from build123d import *
from OCP.BRepFilletAPI import BRepFilletAPI_MakeChamfer

# Parameters (mm, degrees)
DOWELSUPPORT_DEPTH       = 1.905
DOWELSUPPORT_DEPTH_BACK  = 1.27
SKETCH3_R                = 3.81
SKETCH5_W                = 9.525
SKETCH5_H                = 31.75
SLIDERDOWELSUPPORT_DEPTH = 1.27
STRINGDOWELSUPPORT_DEPTH = 1.27
SKETCH9_W                = 6.35
SKETCH9_H                = 3
TABSUPPORT_DEPTH         = 1.27
INTERSUPPORT_DEPTH       = 1.27
DOWELHOLES_DEPTH         = 36.095686544
DOWELHOLES_DEPTH_BACK    = 36.095686544
SKETCH11_R               = 1.600000102
BOSS_EXTRUDE1_START      = -1.27
SKETCH11_2_R             = 1.600000102
BOSS_EXTRUDE1_DEPTH      = 0.254
SKETCH14_W               = 6.35
SKETCH14_H               = 3
TABBASE_DEPTH            = 1.27
SKETCH15_W               = 6.35
SKETCH15_H               = 3
TABDRAFT_DEPTH           = 1.73
TABDRAFT_DRAFT           = 5
TABDRAFT_PROFILE_2_DEPTH = 1.73
TABDRAFT_PROFILE_2_DRAFT = 5
CHAMFER2_SIZE            = 2.54
CUT_EXTRUDE1_DEPTH       = 3
CHAMFER3_SIZE            = 0.508
CHAMFER3_SIZE2           = 1.016


with BuildPart() as part:
    # Sketch3 → DowelSupport (new, two sides: drawn at the far end of the back side and taken through both)
    with BuildSketch(Plane(origin=(0, 0, 0), x_dir=(0, 0, -1), z_dir=(1, 0, 0)).offset(-DOWELSUPPORT_DEPTH_BACK)):
        with Locations((-3.175, 27.23375)):
            Circle(SKETCH3_R)
    extrude(amount=DOWELSUPPORT_DEPTH + DOWELSUPPORT_DEPTH_BACK)



with BuildPart() as body_2:
    # Sketch5 → SliderDowelSupport (new, symmetric)
    with BuildSketch(Plane(origin=(0, 0, 0), x_dir=(0, 0, -1), z_dir=(1, 0, 0))):
        with Locations((-1.5875, 0)):
            Rectangle(SKETCH5_W, SKETCH5_H)
    extrude(amount=SLIDERDOWELSUPPORT_DEPTH, both=True)


with BuildPart() as body_3:
    # Sketch8 → StringDowelSupport (new, symmetric)
    with BuildSketch(Plane(origin=(0, 0, 0), x_dir=(0, 0, -1), z_dir=(1, 0, 0))):
        with BuildLine():
            Line((4.6355, 31.242), (8.0645, 31.242))
            ThreePointArc((8.0645, 31.242), (10.6045, 28.702), (8.0645, 26.162))
            Line((8.0645, 26.162), (4.6355, 26.162))
            ThreePointArc((4.6355, 26.162), (2.0955, 28.702), (4.6355, 31.242))
        make_face()
    extrude(amount=STRINGDOWELSUPPORT_DEPTH, both=True)


with BuildPart() as part_1:
    add(part.part)

    add(body_3.part)  # TabSupport merges body 3
    # Sketch9 → TabSupport (add, symmetric)
    with BuildSketch(Plane(origin=(0, 0, 0), x_dir=(0, 0, -1), z_dir=(1, 0, 0))):
        with Locations((0, 27.94)):
            Rectangle(SKETCH9_W, SKETCH9_H)
        with Locations((12.7, 27.94)):
            Rectangle(SKETCH9_W, SKETCH9_H)
    extrude(amount=TABSUPPORT_DEPTH, both=True)


    add(body_2.part)  # InterSupport merges body 2
    # Sketch10 → InterSupport (add, symmetric)
    with BuildSketch(Plane(origin=(0, 0, 0), x_dir=(0, 0, -1), z_dir=(1, 0, 0))):
        Polygon((-6.35, 15.875), (-5.711088789, 27.374652996), (-3.644260291, 29.730026182), (4.166239709, 31.198276182), (8.657140431, 31.171894192), (15.875, 29.44), (15.875, 26.44), (3.175, 9.525), (3.175, 15.875), align=None)
    extrude(amount=INTERSUPPORT_DEPTH, both=True)

    # Sketch11 → DowelHoles (cut, two sides: drawn at the far end of the back side and taken through both)
    with BuildSketch(Plane(origin=(0, 0, 0), x_dir=(0, 0, -1), z_dir=(1, 0, 0)).offset(-DOWELHOLES_DEPTH_BACK)):
        with Locations((-3.175, 27.23375)):
            Circle(SKETCH11_R)
        with BuildLine():
            Line((6.04239599, 27.94), (6.65760401, 27.94))
            ThreePointArc((6.65760401, 27.94), (9.664500102, 28.702), (6.65760401, 29.464))
            Line((6.65760401, 29.464), (6.04239599, 29.464))
            ThreePointArc((6.04239599, 29.464), (3.035499898, 28.702), (6.04239599, 27.94))
        make_face()
    extrude(amount=DOWELHOLES_DEPTH + DOWELHOLES_DEPTH_BACK, mode=Mode.SUBTRACT)

    # Sketch11<2> → Boss-Extrude1 (add)
    with BuildSketch(Plane(origin=(0, 0, 0), x_dir=(0, 0, -1), z_dir=(1, 0, 0)).offset(BOSS_EXTRUDE1_START)):
        with BuildLine():
            Line((6.04239599, 27.94), (6.65760401, 27.94))
            ThreePointArc((6.65760401, 27.94), (9.664500102, 28.702), (6.65760401, 29.464))
            Line((6.65760401, 29.464), (6.04239599, 29.464))
            ThreePointArc((6.04239599, 29.464), (3.035499898, 28.702), (6.04239599, 27.94))
        make_face()
        with Locations((-3.175, 27.23375)):
            Circle(SKETCH11_2_R)
    extrude(amount=BOSS_EXTRUDE1_DEPTH)

    # Sketch14 → TabBase (add)
    with BuildSketch(Plane.ZY.offset(1.27)):
        with Locations((-12.7, 27.94)):
            Rectangle(SKETCH14_W, SKETCH14_H)
        with Locations((0, 27.94)):
            Rectangle(SKETCH14_W, SKETCH14_H)
    extrude(amount=TABBASE_DEPTH)


with BuildPart() as tabdraft_tool:
    # Sketch15 → TabDraft (with draft: the straight prism first)
    with BuildSketch(Plane.ZY.offset(2.54)):
        with Locations((0, 27.94)):
            Rectangle(SKETCH15_W, SKETCH15_H)
    extrude(amount=TABDRAFT_DEPTH)
    # TabDraft: the draft: its side faces are tilted about the plane it starts from
    tabdraft_sides = [tabdraft_tool.faces().sort_by_distance(p)[0] for p in [
        (-3.405, 27.94, -3.175),
        (-3.405, 26.44, 0),
        (-3.405, 27.94, 3.175),
        (-3.405, 29.44, 0),
    ]]
    draft(tabdraft_sides, Plane.ZY.offset(2.54), TABDRAFT_DRAFT)


with BuildPart() as part_2:
    add(part_1.part)

    # TabDraft: add tabdraft_tool
    add(tabdraft_tool.part)


with BuildPart() as tabdraft_profile_2_tool:
    # Sketch15 → TabDraft profile 2 (with draft: the straight prism first)
    with BuildSketch(Plane.ZY.offset(2.54)):
        with Locations((-12.7, 27.94)):
            Rectangle(SKETCH15_W, SKETCH15_H)
    extrude(amount=TABDRAFT_PROFILE_2_DEPTH)
    # TabDraft profile 2: the draft: its side faces are tilted about the plane it starts from
    tabdraft_profile_2_sides = [tabdraft_profile_2_tool.faces().sort_by_distance(p)[0] for p in [
        (-3.405, 27.94, -15.875),
        (-3.405, 26.44, -12.7),
        (-3.405, 27.94, -9.525),
        (-3.405, 29.44, -12.7),
    ]]
    draft(tabdraft_profile_2_sides, Plane.ZY.offset(2.54), TABDRAFT_PROFILE_2_DRAFT)


with BuildPart() as part_3:
    add(part_2.part)

    # TabDraft profile 2: add tabdraft_profile_2_tool
    add(tabdraft_profile_2_tool.part)

    # Chamfer2
    chamfer2_edges = [part_3.edges().sort_by_distance(p)[0] for p in [
        (1.27, 17.9825, -9.525),
    ]]
    chamfer(chamfer2_edges, length=CHAMFER2_SIZE - 0.0001)  # a hair under: the kernel refuses the full size

    # Mirror1: part across plane


with BuildPart() as part_4:
    add(part_3.part)
    add(part_3.part.mirror(Plane.ZX))

    # Sketch16 → Cut-Extrude1 (cut)
    with BuildSketch(Plane.XY.offset(6.35)):
        Polygon((-1.27, 4.006469684), (-1.27, -4.006469684), (1.27, -2.54), (1.27, 2.54), align=None)
    extrude(amount=-CUT_EXTRUDE1_DEPTH, mode=Mode.SUBTRACT)

    # Chamfer3: one chamfer whose edges measure the first distance from different faces: ONE call of the kernel's chamfer builder (chamfer() names one face for all edges)
    chamfer3_edges_1 = [part_4.edges().sort_by_distance(p)[0] for p in [
        (0, 3.273234842, 6.35),
    ]]
    chamfer3_side_1 = [part_4.faces().sort_by_distance(p)[0] for p in [
        (0.024631688, 9.567006865, 6.35),
    ]]
    chamfer3_edges_2 = [part_4.edges().sort_by_distance(p)[0] for p in [
        (0, -3.273234842, 6.35),
    ]]
    chamfer3_side_2 = [part_4.faces().sort_by_distance(p)[0] for p in [
        (0.024631688, -9.567006865, 6.35),
    ]]
    chamfer3 = BRepFilletAPI_MakeChamfer(part_4.part.solid().wrapped)
    for e in chamfer3_edges_1:
        chamfer3.Add(CHAMFER3_SIZE, CHAMFER3_SIZE2, e.wrapped, chamfer3_side_1[0].wrapped)  # the first distance lies on this face
    for e in chamfer3_edges_2:
        chamfer3.Add(CHAMFER3_SIZE, CHAMFER3_SIZE2, e.wrapped, chamfer3_side_2[0].wrapped)  # the first distance lies on this face
    add(Compound.cast(chamfer3.Shape()), mode=Mode.REPLACE)


solid = part_4.part
Design review of the part built by this model. Coordinates are the model's own, in mm. A direction names the side the tool comes from. Round coordinates to 2 decimals unless told otherwise and drop trailing zeros. Write each loop counter-clockwise with the first axis right and the second up, starting at its lowest first coordinate (ties: lowest second). Pieces come first, ordered by that corner, then holes. Notation, with made-up numbers: M 25,86.25 L 39,86.25 A13 ccw 39,106.25 Z; hole C 71,83.5 d3. An arc over 180 degrees is marked long. One line per item, written item: value. Start each with the question number.
1. To check wall thickness, follow probe 1 along Z at (x, y) = (-1.75, 28.5) (3 decimals); probe 2 along Y at (x, z) = (-1.5, -0.75); probe 3 along Y at (x, z) = (0.25, -3.5). State the ranges of each line that lie inside material, in increasing order. Write a range as from..to.
2. Clearance check with flat-ended pins moving along their axes: P1, Ø2.5, axis at y = 28, z = -7.5, coming from the +X side; P2, Ø1, axis at x = -2, z = -13, coming from the +Y side; P3, Ø2, axis at x = 0.5, y = -9.5, coming from the +Z side. State where each tip first meets the part, or that it passes through.
3. Take a section at C-C on y = 6. State the section outline as (x, z) points (3 decimals), then the cut area to 3 significant figures.
4. For faces 1 (the face through (-3.4, 27.9, -3.1)), 2 (the face through (-3.393, -26.515, -12.744)), 3 (the face through (0, 19.8, -9.3)), 4 (the face through (0.111, -28.761, -3.037)), 5 (the face through (0.02, 3.26, 4.36)), list the 3-axis set-ups (+Z, -Z, +X, -X, +Y, -Y) from which the entire face can be reached by the end or side of a thin tool; tool diameter is ignored.
5. Take a section at B-B on z = -1.75. State the section outline as (x, y) points, then the cut area to 3 significant figures.
6. Take a section at A-A on x = -3.25. State the section outline as (y, z) points, then the cut area to 3 significant figures.
7. Draft analysis for pull direction Z (two halves, no side actions). For faces 6 (the face through (0.018, -30.318, -12.216)), 7 (the face through (-2, 29.44, 0)), 8 (the face through (-2, 28, -3.175)), state which applies: pulls with the +Z half, pulls with the -Z half, needs draft (parallel to the pull), parting line crosses it, or undercut.
Computed:
1. probe 1: z = -15.875..-9.525, -3.175..3.175
1. probe 2: y = -29.44..-26.44, 26.44..29.44
1. probe 3: y = -31.07..-29.83, -27.57..-12.49, 12.49..27.57, 29.83..31.07
2. P1: stops at x = 1.27
2. P2: stops at y = 29.44
2. P3: stops at z = 6.35
3. outline: M -1.27,-3.175 L 1.27,-3.175 L 1.27,6.35 L -1.27,6.35 Z
3. area: 24.2 mm²
4. face 1: -X, +Y, -Y
4. face 2: +Z, -Z, -X
4. face 3: -Z, +X
4. face 4: +X
4. face 5: +Z, -X
5. outline: M -4.27,-29.29 L -2.54,-29.44 L -1.27,-29.44 L -1.27,-30.74 L 1.27,-30.74 L 1.27,30.74 L -1.27,30.74 L -1.27,29.44 L -2.54,29.44 L -4.27,29.29 L -4.27,26.59 L -2.54,26.44 L -1.27,26.44 L -1.27,-26.44 L -2.54,-26.44 L -4.27,-26.59 Z
5. area: 174 mm²
6. outline: M -29.38,-15.81 L -26.5,-15.81 L -26.5,-9.59 L -29.38,-9.59 Z; M -29.38,-3.11 L -26.5,-3.11 L -26.5,3.11 L -29.38,3.11 Z; M 26.5,-15.81 L 29.38,-15.81 L 29.38,-9.59 L 26.5,-9.59 Z; M 26.5,-3.11 L 29.38,-3.11 L 29.38,3.11 L 26.5,3.11 Z
6. area: 71.6 mm²
7. face 6: pulls with the -Z half
7. face 7: needs draft
7. face 8: undercut
